Can you work these out from the model? Positions are in its coordinate system, mm. A direction names the side the tool comes from. Round coordinates to 2 decimals unless told otherwise and drop trailing zeros. Loops run counter-clockwise (first coordinate to the right, second up) from the corner with the lowest first, then second, coordinate; pieces in that order, holes last. Notation, with made-up numbers: M 56,47.5 L 66,47.5 A35 cw 66,81.5 Z; hole C 61.5,82 d3. An arc over 180 degrees is marked long. Answer as CSV lines item,"result".
from build123d import *

# Parameters (mm, degrees)
SKETCH2_W                 = 150
SKETCH2_H                 = 40
BOSS_EXTRUDE1_DEPTH       = 3
BOSS_EXTRUDE2_DEPTH       = 40
SHELL3_T                  = -5
FILLET2_R                 = 5
F_8_0MM_DOWEL_HOLE1_D     = 8
F_8_0MM_DOWEL_HOLE2_D     = 8
F_8_0MM_DOWEL_HOLE2_DEPTH = 5
F_8_0MM_DOWEL_HOLE2_TIP   = 2.403442476
CUT_EXTRUDE1_REACH        = 105.822
SKETCH8_R                 = 3.95
FILLET3_R                 = 3
CUT_EXTRUDE2_REACH        = 110.916
SKETCH9_R                 = 4


with BuildPart() as part:
    # Sketch2 → Boss-Extrude1 (new body)
    with BuildSketch(Plane.ZY.offset(-23)):
        with Locations((-20, 20)):
            Rectangle(SKETCH2_W, SKETCH2_H)
    extrude(amount=BOSS_EXTRUDE1_DEPTH)

    # Sketch3 → Boss-Extrude2 (add)
    with BuildSketch(Plane.XZ):
        Polygon((20, 55), (-20, 0), (20, 0), align=None)
    extrude(amount=-BOSS_EXTRUDE2_DEPTH)

    # Shell3
    shell3_openings = [part.faces().sort_by_distance(p)[0] for p in [
        (0, 20, 27.5),
    ]]
    offset(amount=SHELL3_T, openings=shell3_openings, kind=Kind.INTERSECTION)

    # Fillet2
    # the kernel refuses this fillet: 5 mm, written as the material it takes off along each edge
    with BuildSketch(Plane(origin=(20, -6.365307396, 55), x_dir=(1, 0, 0), z_dir=(0, 1, 0))) as fillet2_piece_1:
        with BuildLine():
            CenterArc((FILLET2_R * 0.509224591703, FILLET2_R), FILLET2_R, 216.027373385, 53.972626615)
            Line((-FILLET2_R * 0.2995114926, FILLET2_R * 0.411828302325), (0, 0))
            Line((0, 0), (FILLET2_R * 0.509224591703, 0))
        make_face()
    extrude(amount=52.730614793, mode=Mode.SUBTRACT)
    with BuildSketch(Plane(origin=(-20, -24.547125578, 0), x_dir=(1, 0, 0), z_dir=(0, 1, 0))) as fillet2_piece_2:
        with BuildLine():
            CenterArc((FILLET2_R * 1.96377004625, -FILLET2_R), FILLET2_R, 90, 126.027373385)
            Line((FILLET2_R * 1.15503396195, -FILLET2_R * 1.58817169768), (0, 0))
            Line((0, 0), (FILLET2_R * 1.96377004625, 0))
        make_face()
    extrude(amount=89.094251156, mode=Mode.SUBTRACT)

    # Ø8.0mm Dowel Hole1 (through all)
    with Locations(Plane.XY.offset(5)):
        with Locations((0, 12.5), (0, 27.5)):
            Hole(F_8_0MM_DOWEL_HOLE1_D / 2)

    # Ø8.0mm Dowel Hole2
    with Locations(Plane.ZY.offset(-18)):
        with Locations((27.5, 20)):
            Hole(F_8_0MM_DOWEL_HOLE2_D / 2, depth=F_8_0MM_DOWEL_HOLE2_DEPTH)
            with Locations((0, 0, -(F_8_0MM_DOWEL_HOLE2_DEPTH + F_8_0MM_DOWEL_HOLE2_TIP / 2))):  # 118° drill point
                Cone(0, F_8_0MM_DOWEL_HOLE2_D / 2, F_8_0MM_DOWEL_HOLE2_TIP, mode=Mode.SUBTRACT)

    # Sketch8 → Cut-Extrude1 (cut, up to next)
    with BuildSketch(Plane.XZ.offset(-35), mode=Mode.PRIVATE) as cut_extrude1_sk1:
        with Locations(Location((10.069403087, 17.720429244, 0), (0, 0, 270))):
            Circle(SKETCH8_R)
    cut_extrude1_tool1 = extrude(cut_extrude1_sk1.sketch, amount=-CUT_EXTRUDE1_REACH, mode=Mode.PRIVATE) & part.part
    add(cut_extrude1_tool1.solids().sort_by_distance((10.069403, 35, 17.720429))[0], mode=Mode.SUBTRACT)

    # Mirror2: part across plane


with BuildPart() as part_1:
    add(part.part)
    add(part.part.mirror(Plane.XY.offset(-20)))

    # Fillet3
    fillet3_edges = [part_1.edges().sort_by_distance(p)[0] for p in [
        (20, 20, 0),
        (20, 20, -40),
    ]]
    fillet(fillet3_edges, radius=FILLET3_R)

    # Sketch9 → Cut-Extrude2 (cut, up to next)
    with BuildSketch(Plane.ZY.offset(-20), mode=Mode.PRIVATE) as cut_extrude2_sk1:
        with Locations((27.5, 20)):
            Circle(SKETCH9_R)
    cut_extrude2_tool1 = extrude(cut_extrude2_sk1.sketch, amount=-CUT_EXTRUDE2_REACH, mode=Mode.PRIVATE) & part_1.part
    # Sketch9 → Cut-Extrude2 (cut, up to next)
    with BuildSketch(Plane.ZY.offset(-20), mode=Mode.PRIVATE) as cut_extrude2_sk2:
        with Locations(Location((-67.5, 20, 0), (0, 0, 180))):
            Circle(SKETCH9_R)
    cut_extrude2_tool2 = extrude(cut_extrude2_sk2.sketch, amount=-CUT_EXTRUDE2_REACH, mode=Mode.PRIVATE) & part_1.part
    add(cut_extrude2_tool1.solids().sort_by_distance((20, 20, 27.5))[0], mode=Mode.SUBTRACT)
    add(cut_extrude2_tool2.solids().sort_by_distance((20, 20, -67.5))[0], mode=Mode.SUBTRACT)


solid = part_1.part
Item 1: If we section it at D-D on y = 3.5: Write out the boundary of the cut face in (x, z), then the cut area to 3 significant figures.
Output:
outline,"M -14.22,-47.94 L 18.5,-92.94 A5 ccw 20,-94.3 L 20,-95 L 23,-95 L 23,55 L 20,55 L 20,54.3 A5 ccw 18.5,52.94 L -14.22,7.94 A5 ccw -10.18,0 L 17,0 A3 cw 20,-3 L 20,-37 A3 cw 17,-40 L -10.18,-40 A5 ccw Z"
area,"2,610 mm2"
Item 2: Will these pins go through, and if not, where does the flat tip stop? pin 1 (10 mm diameter, centred on x = 4.5, z = -75.5, fed in from -Y); pin 2 (0.6 mm diameter, centred on y = 23.5, z = 54.5, fed in from -X); pin 3 (4 mm diameter, centred on x = -2, y = 11, fed in from +Z); pin 4 (1.3 mm diameter, centred on x = 17.5, y = 17.5, fed in from -Z).
Output:
pin 1,"stops at y = 0"
pin 2,"stops at x = 19.83"
pin 3,"stops at z = 5"
pin 4,"stops at z = -92.46"
Item 3: If we section it at B-B on x = 0: State how many separate pieces and enclosed holes the cut face has, then the cut area to 3 significant figures.
Output:
separate pieces,"6"
enclosed holes,"0"
area,"690 mm2"
Item 4: If I drill on line 1 along Y through (x, z) = (0, 3); line 2 along Y through (x, z) = (11, -53.5); line 3 along Y through (x, z) = (22.15, 27.5), over which ranges is the centre line in solid material (lowest first)? Write a range as from..to.
Output:
line 1,"y = 0..8.5, 16.5..23.5, 31.5..40"
line 2,"y = 0..5, 35..40"
line 3,"y = 0..16, 24..40"
Item 5: We'd pull the mould along Y, two halves only. Please class faces 4 (the face through (5, 35, 23)), 5 (the face through (19.1, 20.28, -0.86)), 6 (the face through (5, 5, 23)): released by +Y, released by -Y, zero draft, split by the parting line, or undercut.
Output:
face 4,"undercut"
face 5,"zero draft"
face 6,"undercut"
Item 6: On a 3-axis mill with a long thin cutter (end or side, diameter ignored), from which of +Z, -Z, +X, -X, +Y, -Y can I reach the whole of each face in a straight line? I mean faces 1 (the face through (19.1, 20.28, -39.14)), 2 (the face through (18, 20, -72)), 3 (the face through (6.565, 37.465, -55.898)). Say none if no direction works.
Output:
face 1,"-X, +Y, -Y"
face 2,"-X"
face 3,"+Y"
Item 7: If we section it at A-A on z = -67.5: Write out the boundary of the cut face in (x, y), then the cut area to 3 significant figures.
Output:
outline,"M 0,0 L 23,0 L 23,16 L 18,16 L 18,5 L 0,5 Z; M 0,35 L 18,35 L 18,24 L 23,24 L 23,40 L 0,40 Z"
area,"340 mm2"
